The model under review builds one solid part; all positions refer to its coordinate system, in mm. Face numbers are marked on the shaded views. A direction names the side the tool comes from. Coordinates: 2 decimals unless noted, no trailing zeros. Order: outer loops, then holes, each group sorted by start corner. A loop starts at its lowest first (then second) coordinate and runs counter-clockwise, first axis right, second up.
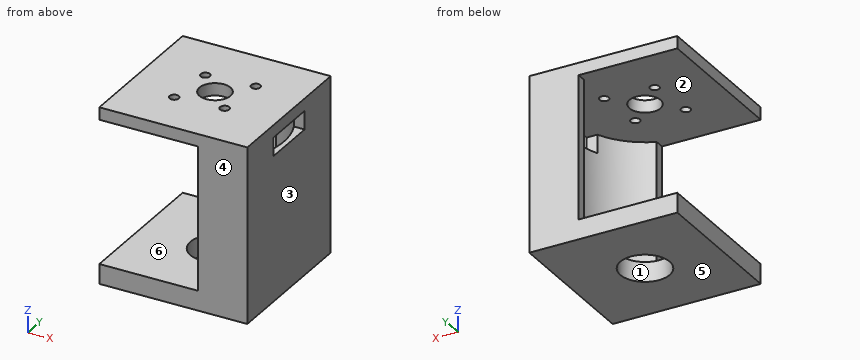
from build123d import *

# Parameters (mm, degrees)
SKETCH2_W           = 38.1
SKETCH2_H           = 38.1
BOSS_EXTRUDE1_DEPTH = 3.175
BOSS_EXTRUDE2_DEPTH = 36.92
SKETCH5_R           = 6.35
BOSS_EXTRUDE3_DEPTH = 5.08
SKETCH8_W           = 4.7625
SKETCH8_H           = 14.2875
CUT_EXTRUDE1_DEPTH  = 60.820669505


with BuildPart() as part:
    # Sketch2 → Boss-Extrude1 (new body)
    with BuildSketch(Plane.XY):
        Rectangle(SKETCH2_W, SKETCH2_H)
        with BuildLine():
            ThreePointArc((5.517514421, 6.717514421), (6.717514421, 5.517514421), (7.917514421, 6.717514421))
            ThreePointArc((7.917514421, 6.717514421), (6.717514421, 7.917514421), (5.517514421, 6.717514421))
        make_face(mode=Mode.SUBTRACT)
        with BuildLine():
            ThreePointArc((4.456854249, -5.656854249), (5.656854249, -6.856854249), (6.856854249, -5.656854249))
            ThreePointArc((6.856854249, -5.656854249), (5.656854249, -4.456854249), (4.456854249, -5.656854249))
        make_face(mode=Mode.SUBTRACT)
        with BuildLine():
            ThreePointArc((-7.917514421, -6.717514421), (-6.717514421, -7.917514421), (-5.517514421, -6.717514421))
            ThreePointArc((-5.517514421, -6.717514421), (-6.717514421, -5.517514421), (-7.917514421, -6.717514421))
        make_face(mode=Mode.SUBTRACT)
        with BuildLine():
            ThreePointArc((-6.856854249, 5.656854249), (-5.656854249, 4.456854249), (-4.456854249, 5.656854249))
            ThreePointArc((-4.456854249, 5.656854249), (-5.656854249, 6.856854249), (-6.856854249, 5.656854249))
        make_face(mode=Mode.SUBTRACT)
        with BuildLine():
            ThreePointArc((0, -4), (4, 0), (0, 4))
            ThreePointArc((0, 4), (-4, 0), (0, -4))
        make_face(mode=Mode.SUBTRACT)
    extrude(amount=BOSS_EXTRUDE1_DEPTH)

    # Sketch3 → Boss-Extrude2 (add)
    with BuildSketch(Plane(origin=(0, 0, 0), x_dir=(-1, 0, 0), z_dir=(0, 0, -1))):
        with BuildLine():
            Line((-19.05, -19.05), (-6.35, -19.05))
            Line((-6.35, -19.05), (-6.35, -16.607404975))
            ThreePointArc((-6.35, -16.607404975), (-17.78, 0), (-6.35, 16.607404975))
            Line((-6.35, 16.607404975), (-6.35, 19.05))
            Line((-6.35, 19.05), (-19.05, 19.05))
            Line((-19.05, 19.05), (-19.05, -19.05))
        make_face()
    extrude(amount=BOSS_EXTRUDE2_DEPTH)

    # Sketch5 → Boss-Extrude3 (add)
    # profile 1 of 3: a face of its own
    with BuildSketch(Plane(origin=(0, 0, -36.92), x_dir=(-1, 0, 0), z_dir=(0, 0, -1))):
        with BuildLine():
            Line((-6.35, -19.05), (19.05, -19.05))
            Line((19.05, -19.05), (19.05, 19.05))
            Line((19.05, 19.05), (-6.35, 19.05))
            Line((-6.35, 19.05), (-6.35, 16.607404975))
            ThreePointArc((-6.35, 16.607404975), (-17.78, 0), (-6.35, -16.607404975))
            Line((-6.35, -16.607404975), (-6.35, -19.05))
        make_face()
        with BuildLine():
            ThreePointArc((-14, 0), (0, 14), (14, 0))
            ThreePointArc((14, 0), (0, -14), (-14, 0))
        make_face(mode=Mode.SUBTRACT)
    # profile 2 of 3: a face of its own
    with BuildSketch(Plane(origin=(0, 0, -36.92), x_dir=(-1, 0, 0), z_dir=(0, 0, -1))):
        with BuildLine():
            ThreePointArc((14, 0), (0, 14), (-14, 0))
            ThreePointArc((-14, 0), (0, -14), (14, 0))
        make_face()
        Circle(SKETCH5_R, mode=Mode.SUBTRACT)
    # profile 3 of 3: a face of its own
    with BuildSketch(Plane(origin=(0, 0, -36.92), x_dir=(-1, 0, 0), z_dir=(0, 0, -1))):
        with BuildLine():
            Line((-6.35, -19.05), (-6.35, -16.607404975))
            ThreePointArc((-6.35, -16.607404975), (-17.78, 0), (-6.35, 16.607404975))
            Line((-6.35, 16.607404975), (-6.35, 19.05))
            Line((-6.35, 19.05), (-19.05, 19.05))
            Line((-19.05, 19.05), (-19.05, -19.05))
            Line((-19.05, -19.05), (-6.35, -19.05))
        make_face()
    extrude(amount=BOSS_EXTRUDE3_DEPTH)

    # Sketch8 → Cut-Extrude1 (cut, through all)
    with BuildSketch(Plane(origin=(19.05, 0, 0), x_dir=(0, 0, -1), z_dir=(1, 0, 0))):
        with Locations((2.38125, 0)):
            Rectangle(SKETCH8_W, SKETCH8_H)
    extrude(amount=-CUT_EXTRUDE1_DEPTH, mode=Mode.SUBTRACT)


solid = part.part
(1) Consider section C-C (z = -4). Give the boundary of the cut face in (x, y).
(2) Consider section B-B (x = -14). Give the boundary of the cut face in (y, z) (3 decimals), then the cut area to 3 significant figures.
(3) Tool access review of the marked faces 1, 2 and 3: name each direction out of +Z, -Z, +X, -X, +Y, -Y from which nothing blocks a thin tool from reaching the whole face with its end or side.
(4) Consider section D-D (x = 0). Give the boundary of the cut face in (y, z) (3 decimals).
(5) Consider section A-A (y = 0). Give the number of separate pieces and of enclosed holes in the cut face, then the cut area to 3 significant figures.
(6) Insertion check: pin 1 Ø1.9 at (x, y) = (-6.72, -6.72) entering from +Z; pin 2 Ø2 at (y, z) = (-18.5, -15.5) entering from -X; pin 3 Ø0.7 at (y, z) = (18, -10.5) entering from -X. Each pin has a flat end and moves straight along its axis. Give the tip position at first contact, or say it passes through.
(7) Wall thickness on line 1 (Z direction, x = 10, y = -8.5) (3 decimals); line 2 (X direction, y = 0, z = 1.1); line 3 (Y direction, x = -2.5, z = -37.5): over which ranges is each line inside the solid? List them lowest first.
(8) The part is to be moulded in two halves that separate along Z. For the marked faces 4, 5 and 6, say which applies: +Z half, -Z half, draft (parallel to the pull), parting line (faces both ways), or undercut.
Findings:
1. outline: (6.35, -19.05) - (19.05, -19.05) - (19.05, -7.14) - (16.28, -7.14) arc R17.78 cw to (6.35, -16.61) - close; (6.35, 16.61) arc R17.78 cw to (16.28, 7.14) - (19.05, 7.14) - (19.05, 19.05) - (6.35, 19.05) - close
2. outline: (-19.05, -42) - (19.05, -42) - (19.05, -36.92) - (-19.05, -36.92) - close; (-19.05, 0) - (19.05, 0) - (19.05, 3.175) - (-19.05, 3.175) - close
2. area: 315 mm2
3. face 1: -Z
3. face 2: -X
3. face 3: +Z, -Z, +X, +Y, -Y
4. outline: (-19.05, -42) - (-6.35, -42) - (-6.35, -36.92) - (-19.05, -36.92) - close; (-19.05, 0) - (-4, 0) - (-4, 3.175) - (-19.05, 3.175) - close; (4, 0) - (19.05, 0) - (19.05, 3.175) - (4, 3.175) - close; (6.35, -42) - (19.05, -42) - (19.05, -36.92) - (6.35, -36.92) - close
5. separate pieces: 4
5. enclosed holes: 0
5. area: 265 mm2
6. pin 1: stops at z = -36.92
6. pin 2: stops at x = 6.35
6. pin 3: stops at x = 6.35
7. line 1: z = -42 to -36.92, 0 to 3.175
7. line 2: x = -19.05 to -4, 4 to 19.05
7. line 3: y = -19.05 to -5.84, 5.84 to 19.05
8. face 4: draft
8. face 5: -Z half
8. face 6: undercut
